Geometry check sheet. Reference: the model listing, model coordinates, mm. A direction names the side the tool comes from. Round coordinates to 2 decimals unless told otherwise and drop trailing zeros. Write each loop counter-clockwise with the first axis right and the second up, starting at its lowest first coordinate (ties: lowest second). Pieces come first, ordered by that corner, then holes. Notation, with made-up numbers: (22, -16.75) - (48, -16.75) arc R18 ccw to (48, 7.25) - close; hole circle Ø9 at (20, 54). An arc over 180 degrees is marked (long way). Return JSON: item names as keys, results as strings.
```python
from build123d import *

# Parameters (mm, degrees)
SKETCH1_R           = 2.45
SKETCH1_R_2         = 1.6
BOSS_EXTRUDE1_DEPTH = 19
SKETCH2_R           = 7.5
BOSS_EXTRUDE2_DEPTH = 3
CUT_EXTRUDE1_REACH  = 26.423
SKETCH3_R           = 1.6
CUT_EXTRUDE2_DEPTH  = 2.5


with BuildPart() as part:
    # Sketch1 → Boss-Extrude1 (new body)
    with BuildSketch(Plane(origin=(0, 0, 0), x_dir=(1, 0, 0), z_dir=(0, 1, 0))):
        with Locations(Location((0, 0, 0), (0, 0, 270))):
            Circle(SKETCH1_R)
        with Locations(Location((0, 0, 0), (0, 0, 270))):
            Circle(SKETCH1_R_2, mode=Mode.SUBTRACT)
    extrude(amount=BOSS_EXTRUDE1_DEPTH)

    # Sketch2 → Boss-Extrude2 (add)
    with BuildSketch(Plane(origin=(0, 19, 0), x_dir=(1, 0, 0), z_dir=(0, 1, 0))):
        with Locations(Location((0, 0, 0), (0, 0, 270))):
            Circle(SKETCH2_R)
    extrude(amount=BOSS_EXTRUDE2_DEPTH)

    # Sketch3 → Cut-Extrude1 (cut, up to next)
    with BuildSketch(Plane(origin=(0, 22, 0), x_dir=(1, 0, 0), z_dir=(0, 1, 0)), mode=Mode.PRIVATE) as cut_extrude1_sk1:
        with Locations(Location((0, 0, 0), (0, 0, 270))):
            Circle(SKETCH3_R)
    cut_extrude1_tool1 = extrude(cut_extrude1_sk1.sketch, amount=-CUT_EXTRUDE1_REACH, mode=Mode.PRIVATE) & part.part
    add(cut_extrude1_tool1.solids().sort_by_distance((0, 22, 0))[0], mode=Mode.SUBTRACT)

    # Sketch4 → Cut-Extrude2 (cut)
    with BuildSketch(Plane(origin=(0, 22, 0), x_dir=(1, 0, 0), z_dir=(0, 1, 0))):
        Polygon((3.233161507, 0), (1.616580754, 2.8), (-1.616580754, 2.8), (-3.233161507, 0), (-1.616580754, -2.8), (1.616580754, -2.8), align=None)
    extrude(amount=-CUT_EXTRUDE2_DEPTH, mode=Mode.SUBTRACT)


solid = part.part
```
(1) Section check C-C, the plane z = 3.25. Enter the section's corners in (x, y).
Response values:
{"outline": "(-6.76, 19) - (6.76, 19) - (6.76, 22) - (-6.76, 22) - close"}
(2) Section check A-A, the plane x = 0. Enter the section's corners in (y, z).
Response values:
{"outline": "(0, -2.45) - (19, -2.45) - (19, -7.5) - (22, -7.5) - (22, -2.8) - (19.5, -2.8) - (19.5, -1.6) - (0, -1.6) - close; (0, 1.6) - (19.5, 1.6) - (19.5, 2.8) - (22, 2.8) - (22, 7.5) - (19, 7.5) - (19, 2.45) - (0, 2.45) - close"}
(3) Material ranges on line 1 along X through (y, z) = (9.75, 0); line 2 along Y through (x, z) = (-3.5, -6.25); line 3 along Y through (x, z) = (-1.5, 1.75), recorded low to high. Write a range as [from, to].
Response values:
{"line 1": "x = [-2.45, -1.6], [1.6, 2.45]", "line 2": "y = [19, 22]", "line 3": "y = [0, 19.5]"}
(4) Section check B-B, the plane y = 16. Enter the section's corners in (x, z).
Response values:
{"outline": "circle Ø4.9 at (0, 0); hole circle Ø3.2 at (0, 0)"}
(5) Access from +Z, -Z, +X, -X, +Y, -Y to the whole of each face (thin tool, end or side, straight path). Record for faces 1 (the face through (-0.97, 9.89, -1.27)), 2 (the face through (0, 21, 2.8)).
Response values:
{"face 1": "+Y, -Y", "face 2": "+Y"}
(6) Gauge pin test, flat ends, axial feed: pin 1 (1.5 mm diameter, centred on x = 2, y = 5, fed in from +Z); pin 2 (3 mm diameter, centred on y = 9, z = 3.5, fed in from +X). Record the tip position at first contact, or that the pin passes through.
Response values:
{"pin 1": "stops at z = 2.11", "pin 2": "stops at x = 1.42"}
(7) Section check D-D, the plane x = -4.25. Enter the section's corners in (y, z).
Response values:
{"outline": "(19, -6.18) - (22, -6.18) - (22, 6.18) - (19, 6.18) - close"}
(8) Release check for a two-part mould opening along X. For faces 3 (the face through (-2.414, 20.768, -1.42)), 4 (the face through (0.736, 9.367, 2.337)), 5 (the face through (2, 19, -2)) record: pulls with the +X half, pulls with the -X half, needs draft (parallel to the pull), parting line crosses it, or undercut.
Response values:
{"face 3": "undercut", "face 4": "parting line crosses it", "face 5": "needs draft"}
